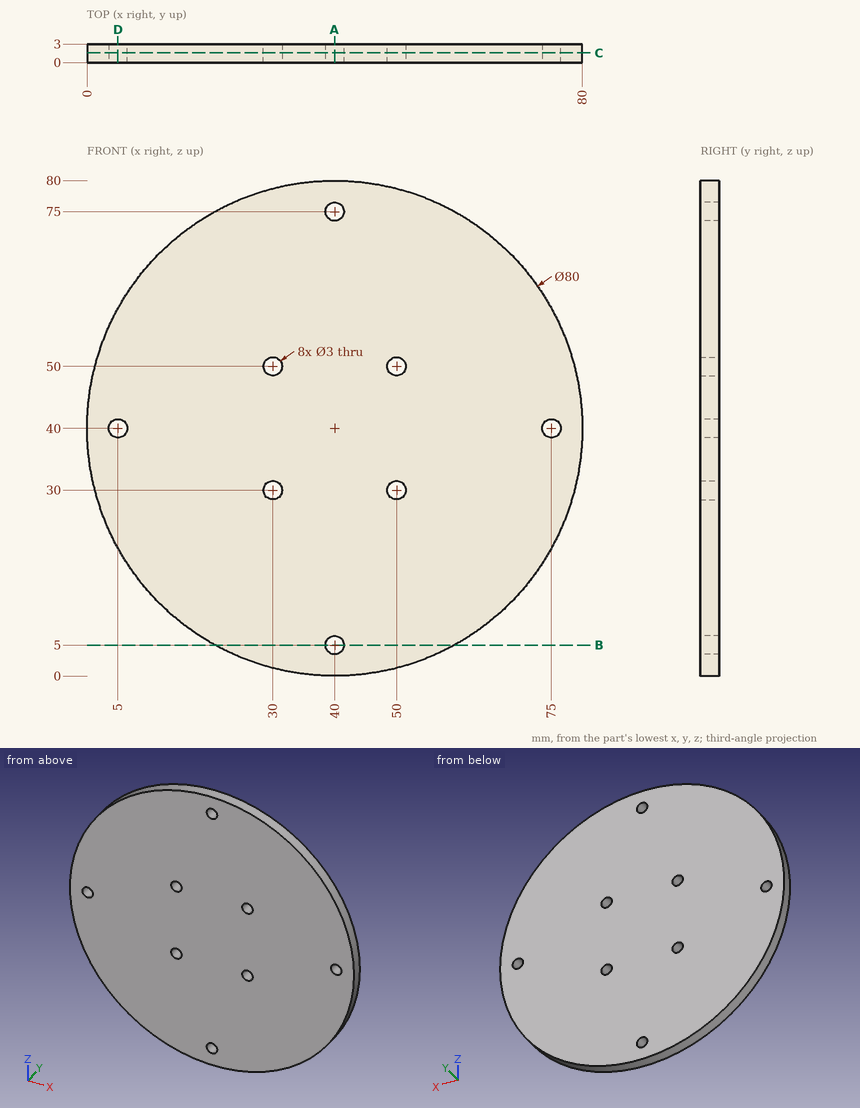
Could you check a few things on this drawing? It's one solid part, dimensions in mm from its lowest x, y, z. Round coordinates to 2 decimals unless told otherwise and drop trailing zeros. Write each loop counter-clockwise with the first axis right and the second up, starting at its lowest first coordinate (ties: lowest second). Pieces come first, ordered by that corner, then holes. Notation, with made-up numbers: M -14.75,83.5 L 16.25,83.5 A21 ccw 16.25,114.5 Z; hole C -0.5,58.5 d5. An arc over 180 degrees is marked long. Answer as CSV lines item,"result". Start each with the question number.
1. I'm going to push flat-ended pins straight in: pin 1 Ø1.5 at (y, z) = (2, 38.5) entering from +X; pin 2 Ø1 at (y, z) = (1.5, 58.5) entering from -X. Where does each tip first touch, or does it pass through?
2. Suppose I cut it at B-B on z = 5. Write out the boundary of the cut face in (x, y), then the cut area to 3 significant figures.
3. Suppose I cut it at A-A on x = 40. Write out the boundary of the cut face in (y, z), then the cut area to 3 significant figures.
4. Suppose I cut it at C-C on y = 1.55. Count the separate pieces of the cut face and the enclosed holes in it, then the cut area to 3 significant figures.
5. I need wall thicknesses on probe 1 along Z at (x, y) = (40, 1.55); probe 2 along X at (y, z) = (1.75, 50). Which ranges of each line are inside material? Lowest first, please.
6. Suppose I cut it at D-D on x = 5. Write out the boundary of the cut face in (y, z), then the cut area to 3 significant figures.
Check result:
1,pin 1,"stops at x = 79.99"
1,pin 2,"stops at x = 4.28"
2,outline,"M 20.64,0 L 38.5,0 L 38.5,3 L 20.64,3 Z; M 41.5,0 L 59.36,0 L 59.36,3 L 41.5,3 Z"
2,area,"107 mm2"
3,outline,"M 0,0 L 3,0 L 3,3.5 L 0,3.5 Z; M 0,6.5 L 3,6.5 L 3,73.5 L 0,73.5 Z; M 0,76.5 L 3,76.5 L 3,80 L 0,80 Z"
3,area,"222 mm2"
4,separate pieces,"1"
4,enclosed holes,"8"
4,area,"4,970 mm2"
5,probe 1,"z = 0 to 3.5, 6.5 to 73.5, 76.5 to 80"
5,probe 2,"x = 1.27 to 28.5, 31.5 to 48.5, 51.5 to 78.73"
6,outline,"M 0,20.64 L 3,20.64 L 3,38.5 L 0,38.5 Z; M 0,41.5 L 3,41.5 L 3,59.36 L 0,59.36 Z"
6,area,"107 mm2"
